from build123d import *

# Parameters (mm, degrees)
BOSS_EXTRUDE1_DEPTH = 2
SKETCH2_R           = 6.4
CUT_EXTRUDE1_DEPTH  = 1
CUT_EXTRUDE4_REACH  = 17.225
SKETCH8_W           = 4.983499023
SKETCH8_H           = 1.601104922
BOSS_EXTRUDE4_DEPTH = 0.01
SKETCH9_W           = 1.2
SKETCH9_H           = 4.7
BOSS_EXTRUDE5_DEPTH = 0.3


with BuildPart() as part:
    # Sketch1 → Boss-Extrude1 (new body)
    with BuildSketch(Plane(origin=(0, 0, 0), x_dir=(1, 0, 0), z_dir=(0, 1, 0))):
        Polygon((-6.75, 6.75), (6.75, 6.75), (6.75, -5.061772225), (5.061772225, -6.75), (-5.061772225, -6.75), (-6.75, -5.061772225), align=None)
    extrude(amount=BOSS_EXTRUDE1_DEPTH)

    # Sketch2 → Cut-Extrude1 (cut)
    with BuildSketch(Plane(origin=(0, 2, 0), x_dir=(1, 0, 0), z_dir=(0, 1, 0))):
        with Locations(Location((0, 0, 0), (0, 0, 270))):
            Circle(SKETCH2_R)
    extrude(amount=-CUT_EXTRUDE1_DEPTH, mode=Mode.SUBTRACT)

    # Cut-Extrude4: up to this face of the body (flat: up to its plane)
    cut_extrude4_end = Plane(part.part.faces().sort_by_distance((6.75, 1, -0.844113887))[0])
    # Sketch8 → Cut-Extrude4 (cut, up to the picked face)
    with BuildSketch(Plane.ZY.offset(6.75), mode=Mode.PRIVATE) as cut_extrude4_sk1:
        with Locations((3.408264651, 2.017914887)):
            Rectangle(SKETCH8_W, SKETCH8_H)
    cut_extrude4_tool1 = split(extrude(cut_extrude4_sk1.sketch, amount=-CUT_EXTRUDE4_REACH, mode=Mode.PRIVATE), bisect_by=cut_extrude4_end, keep=Keep.BOTH, mode=Mode.PRIVATE)
    add(cut_extrude4_tool1.solids().sort_by(Axis((-6.75, 2.017915, 3.408265), (1, 0, 0)))[0], mode=Mode.SUBTRACT)

    # Sketch5 → Revolve1 (revolve)
    with BuildSketch(Plane.XY, mode=Mode.PRIVATE) as revolve1_sk:
        with BuildLine():
            Line((0, 0), (-6.4, 0))
            Line((-6.4, 0), (-6.4, 1.5))
            ThreePointArc((-6.4, 1.5), (-6.3, 1.6), (-6.4, 1.7))
            Line((-6.4, 1.7), (-6.4, 12.65))
            ThreePointArc((-6.4, 12.65), (-6.356066017, 12.756066017), (-6.25, 12.8))
            Line((-6.25, 12.8), (0, 12.8))
            Line((0, 12.8), (0, 0))
        make_face()
    revolve(revolve1_sk.sketch.rotate(Axis((0, 12.8, 0), (0, -1, 0)), 270), axis=Axis((0, 12.8, 0), (0, -1, 0)))

    # Sketch6 → Boss-Extrude4 (add)
    with BuildSketch(Plane(origin=(0, 12.8, 0), x_dir=(1, 0, 0), z_dir=(0, 1, 0))):
        with BuildLine():
            Line((-5.525359589, 2.921113044), (5.525359589, 2.921113044))
            ThreePointArc((5.525359589, 2.921113044), (0, 6.25), (-5.525359589, 2.921113044))
        make_face()
    extrude(amount=BOSS_EXTRUDE4_DEPTH)

    # Sketch9 → Boss-Extrude5 (add)
    with BuildSketch(Plane.XZ):
        with Locations((0, -4.55)):
            Rectangle(SKETCH9_W, SKETCH9_H)
        with Locations((0, 4.55)):
            Rectangle(SKETCH9_W, SKETCH9_H)
    extrude(amount=BOSS_EXTRUDE5_DEPTH)


solid = part.part
Read the model definition and answer for the solid it produces. Units are mm, in the model's axes. A direction names the side the tool comes from. Coordinates: 2 decimals unless noted, no trailing zeros. Loops run counter-clockwise (first coordinate to the right, second up) from the corner with the lowest first, then second, coordinate; pieces in that order, holes last. Notation, with made-up numbers: (-3, 57) - (44, 57) arc R35 ccw to (44, 89) - close; hole circle Ø3 at (41, 17.25). An arc over 180 degrees is marked (long way). Answer in a Markdown table with one row per item.
Q1. Find section C-C on y = 8. Write down the section's boundary in (x, z), plus the area to 3 significant figures.
Here are the results:
| item | result |
|---|---|
| outline | circle Ø12.8 at (0, 0) |
| area | 129 mm^2 |
Q2. Find section B-B on z = 0. Write down the section's boundary in (x, y), plus the area to 3 significant figures.
Here are the results:
| item | result |
|---|---|
| outline | (-6.75, 0) - (6.75, 0) - (6.75, 2) - (6.4, 2) - (6.4, 12.65) arc R0.15 ccw to (6.25, 12.8) - (-6.25, 12.8) arc R0.15 ccw to (-6.4, 12.65) - (-6.4, 2) - (-6.75, 2) - close; hole (-6.4, 1.5) arc R0.1 ccw to (-6.4, 1.7) - close; hole (6.4, 1.5) - (6.4, 1.7) arc R0.1 ccw to start |
| area | 165 mm^2 |
Q3. Straight lines are drawn through the part: line 1 along Y through (x, z) = (-3.5, 5.5); line 2 along Y through (x, z) = (5.25, -5.25); line 3 along X through (y, z) = (11.25, -4). For each, find the intervals that lie inside material, in ascending order. Write a range as [from, to].
Here are the results:
| item | result |
|---|---|
| line 1 | y = [0, 1.22] |
| line 2 | y = [0, 2] |
| line 3 | x = [-5, 5] |
Q4. Given P1, Ø1.5, axis at x = 1, y = 4, coming from the -Z side; P2, Ø1.5, axis at x = -2.5, y = 4.5, coming from the +Z side; P3, Ø1, axis at x = -1, y = 1, coming from the +Z side, each flat-ended and moving along its own axis, determine where each tip first touches the part or whether it passes through.
Here are the results:
| item | result |
|---|---|
| P1 | stops at z = -6.4 |
| P2 | stops at z = 6.16 |
| P3 | stops at z = 6.75 |
Q5. Find section A-A on x = 0. Count the separate pieces of the cut face and the enclosed holes in it, plus the area to 3 significant figures.
Here are the results:
| item | result |
|---|---|
| separate pieces | 1 |
| enclosed holes | 2 |
| area | 168 mm^2 |
Q6. For faces 1 (the flat face through (6, 1.217, 4)), 2 (the flat face through (0, -0.3, 5)), 3 (the cylindrical face through (3.89, 7.25, -5.08)), determine the directions among +Z, -Z, +X, -X, +Y, -Y from which every point of the face is accessible in a straight line to the end or side of a thin tool.
Here are the results:
| item | result |
|---|---|
| face 1 | +X, +Y |
| face 2 | +Z, -Z, +X, -X, -Y |
| face 3 | +Y |
Q7. The mould has two halves that part along Z. Classify faces 4 (the flat face through (0.1, 2, 6.6)), 5 (the flat face through (0, 1, -6.75)), 6 (the flat face through (0, 1, 6.75)), 7 (the flat face through (-6, 1.217, 4)): pulls with the +Z half, pulls with the -Z half, needs draft (parallel to the pull), parting line crosses it, or undercut.
Here are the results:
| item | result |
|---|---|
| face 4 | needs draft |
| face 5 | pulls with the -Z half |
| face 6 | pulls with the +Z half |
| face 7 | undercut |
